Here's the drawing with two shaded views (mm, measured from the low corner). I have some questions. Give positions to 0.01 mm unless a question says otherwise; leave off trailing zeros. Write each loop counter-clockwise with the first axis right and the second up, starting at its lowest first coordinate (ties: lowest second). Pieces come first, ordered by that corner, then holes. Notation, with made-up numbers: M 48,84 L 68,84 A20 ccw 68,100 Z; hole C 64,69 d2. An arc over 180 degrees is marked long. Answer as CSV lines item,"result". Start each with the question number.
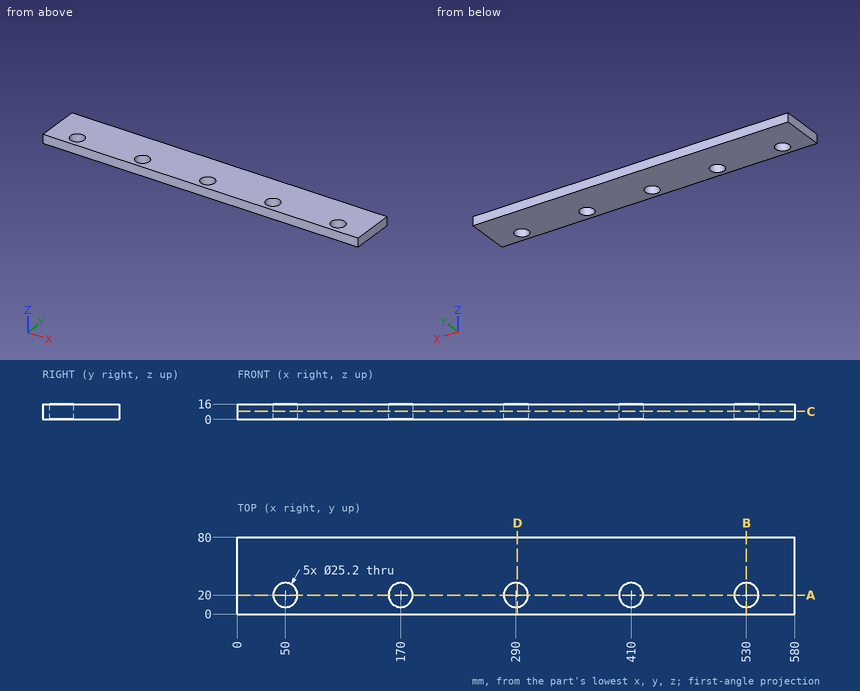
1. Imagine slicing it at B-B, the plane x = 530. Please give me the cut outline in (y, z), plus the area to 3 significant figures.
2. Imagine slicing it at C-C, the plane z = 8.25. Please give me the cut outline in (x, y).
3. Imagine slicing it at A-A, the plane y = 20. Please give me the cut outline in (x, z), plus the area to 3 significant figures.
4. Please list where these lines run through material, in increasing order: line 1 (Y direction, x = 410, z = 11.25); line 2 (X direction, y = 10, z = 5.5); line 3 (X direction, y = 24, z = 2.75).
5. Imagine slicing it at D-D, the plane x = 291.5. Please give me the cut outline in (y, z), plus the area to 3 significant figures.
Solutions:
1,outline,"M 0,0 L 7.4,0 L 7.4,16 L 0,16 Z; M 32.6,0 L 80,0 L 80,16 L 32.6,16 Z"
1,area,"877 mm²"
2,outline,"M 0,0 L 580,0 L 580,80 L 0,80 Z; hole C 50,20 d25.2; hole C 170,20 d25.2; hole C 290,20 d25.2; hole C 410,20 d25.2; hole C 530,20 d25.2"
3,outline,"M 0,0 L 37.4,0 L 37.4,16 L 0,16 Z; M 62.6,0 L 157.4,0 L 157.4,16 L 62.6,16 Z; M 182.6,0 L 277.4,0 L 277.4,16 L 182.6,16 Z; M 302.6,0 L 397.4,0 L 397.4,16 L 302.6,16 Z; M 422.6,0 L 517.4,0 L 517.4,16 L 422.6,16 Z; M 542.6,0 L 580,0 L 580,16 L 542.6,16 Z"
3,area,"7,260 mm²"
4,line 1,"0 to 7.4, 32.6 to 80"
4,line 2,"0 to 42.33, 57.67 to 162.33, 177.67 to 282.33, 297.67 to 402.33, 417.67 to 522.33, 537.67 to 580"
4,line 3,"0 to 38.05, 61.95 to 158.05, 181.95 to 278.05, 301.95 to 398.05, 421.95 to 518.05, 541.95 to 580"
5,outline,"M 0,0 L 7.49,0 L 7.49,16 L 0,16 Z; M 32.51,0 L 80,0 L 80,16 L 32.51,16 Z"
5,area,"880 mm²"
